from build123d import *

# Parameters (mm, degrees)
F0_R     = 2.5
F1_DEPTH = 15
F2_R     = 2


with BuildPart() as f1:
    # F0 (on Top) → F1 (new body)
    with BuildSketch(Plane.XY):
        with BuildLine():
            Line((0, 30), (0, 0))
            Line((0, 0), (10, 0))
            Line((10, 0), (10, 10))
            ThreePointArc((10, 10), (20, 20), (10, 30))
            Line((10, 30), (0, 30))
        make_face()
        with Locations((10, 20)):
            Circle(F0_R, mode=Mode.SUBTRACT)
    extrude(amount=F1_DEPTH)

    # F2
    f2_edges = [f1.edges().sort_by_distance(p)[0] for p in [
        (5, 0, 15),
        (10, 5, 15),
        (20, 20, 15),
        (0, 15, 15),
        (0, 15, 0),
        (10, 10, 7.5),
        (10, 30, 7.5),
        (20, 20, 0),
        (7.5, 20, 0),
        (5, 0, 0),
        (0, 0, 7.5),
        (10, 0, 7.5),
        (0, 30, 7.5),
        (12.5, 20, 7.5),
        (7.5, 20, 15),
        (5, 30, 15),
        (5, 30, 0),
        (10, 5, 0),
    ]]
    fillet(f2_edges, radius=F2_R)


solid = f1.part
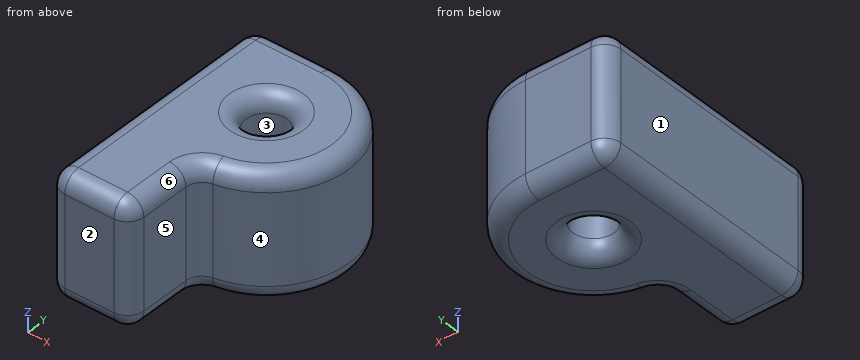
Read the model definition and answer for the solid it produces. Units are mm, in the model's axes. Face numbers are marked on the shaded views. A direction names the side the tool comes from. Give positions to 0.01 mm unless a question says otherwise; leave off trailing zeros. Write each loop counter-clockwise with the first axis right and the second up, starting at its lowest first coordinate (ties: lowest second). Pieces come first, ordered by that corner, then holes. Notation, with made-up numbers: (-21, 69) - (14, 69) arc R23 ccw to (14, 81) - close; hole circle Ø1 at (15, 30). An arc over 180 degrees is marked (long way). Answer in a Markdown table with one row per item. Add a question column.
Item 1: Section D-D, the plane x = 1.25 is taken. Write down the section's boundary in (y, z), and give its area (3 significant figures).
Item 2: Flat-ended cylindrical pins translate along their axes: P1, Ø3, axis at y = 5.5, z = 9.5, coming from the +X side; P2, Ø8, axis at x = 10, y = 20, coming from the +Z side; P3, Ø1.5, axis at y = 18.5, z = 6.5, coming from the +X side. Find the tip coordinate at first contact, or state that the pin passes through.
Item 3: Section B-B, the plane z = 10 is taken. Write down the section's boundary in (x, y), and give its area (3 significant figures).
Item 4: Find the intervals of material crossed by L1, parallel to X at y = 7, z = 10.75; L2, parallel to Y at x = 11, z = 3.25; L3, parallel to X at y = 16, z = 14.25, in increasing order.
Item 5: A tool of negligible diameter and unlimited length cuts with its end or side. For the marked faces 4, 5 and 6, from which of +Z, -Z, +X, -X, +Y, -Y can it reach the whole face along a straight path? Write none if from no direction.
Item 6: Section C-C, the plane y = 4.5 is taken. Write down the section's boundary in (x, z).
Item 7: Determine the mould class of the marked faces 1, 2 and 3 for opening direction Y: pulls with the +Y half, pulls with the -Y half, needs draft (parallel to the pull), parting line crosses it, or undercut.
Item 8: Section A-A, the plane y = 20 is taken. Write down the section's boundary in (x, z), and give its area (3 significant figures).
Recorded:
| question | item | result |
|---|---|---|
| 1 | outline | (0.15, 2) arc R1.85 ccw to (2, 0.15) - (28, 0.15) arc R1.85 ccw to (29.85, 2) - (29.85, 13) arc R1.85 ccw to (28, 14.85) - (2, 14.85) arc R1.85 ccw to (0.15, 13) - close |
| 1 | area | 434 mm2 |
| 2 | P1 | stops at x = 10 |
| 2 | P2 | stops at z = 14.94 |
| 2 | P3 | stops at x = 19.97 |
| 3 | outline | (0, 2) arc R2 ccw to (2, 0) - (8, 0) arc R2 ccw to (10, 2) - (10, 8.17) arc R2 cw to (11.67, 10.14) arc R10 ccw to (10, 30) - (2, 30) arc R2 ccw to (0, 28) - close; hole circle Ø5 at (10, 20) |
| 3 | area | 436 mm2 |
| 4 | L1 | x = 0 to 10 |
| 4 | L2 | y = 9.9 to 17.71, 22.29 to 29.95 |
| 4 | L3 | x = 0.44 to 18.68 |
| 5 | face 4 | +Z, -Z, +X |
| 5 | face 5 | +Z, -Z, +X, -Y |
| 5 | face 6 | +Z, +X, -Y |
| 6 | outline | (0, 2) arc R2 ccw to (2, 0) - (8, 0) arc R2 ccw to (10, 2) - (10, 13) arc R2 ccw to (8, 15) - (2, 15) arc R2 ccw to (0, 13) - close |
| 7 | face 1 | needs draft |
| 7 | face 2 | pulls with the -Y half |
| 7 | face 3 | undercut |
| 8 | outline | (0, 2) arc R2 ccw to (2, 0) - (5.5, 0) arc R2 ccw to (7.5, 2) - (7.5, 13) arc R2 ccw to (5.5, 15) - (2, 15) arc R2 ccw to (0, 13) - close; (12.5, 2) arc R2 ccw to (14.5, 0) - (18, 0) arc R2 ccw to (20, 2) - (20, 13) arc R2 ccw to (18, 15) - (14.5, 15) arc R2 ccw to (12.5, 13) - close |
| 8 | area | 218 mm2 |
